```python
from build123d import *

# Parameters (mm, degrees)
F0_W     = 100
F0_H     = 200
F1_DEPTH = 30
F3_DEPTH = 10
F4_R     = 45
F4_R_2   = 5
F4_R_3   = 30
F5_DEPTH = 10
F6_DEPTH = 27
F7_DEPTH = 32
F9_DEPTH = 10


with BuildPart() as f1:
    # F0 (on Front) → F1 (new body)
    with BuildSketch(Plane.XZ):
        with Locations((50, -100)):
            Rectangle(F0_W, F0_H)
    extrude(amount=F1_DEPTH)

    # F2 (on face) → F3 (join)
    with BuildSketch(Plane(origin=(0, 0, 0), x_dir=(-1, 0, 0), z_dir=(0, 1, 0))):
        with BuildLine():
            ThreePointArc((-38.8196601125, -8.1037424163), (-43.876275643, -4.4106784786), (-50, -3.1037424163))
            ThreePointArc((-50, -3.1037424163), (-56.123724357, -4.4106784786), (-61.1803398875, -8.1037424163))
            Line((-61.1803398875, -8.1037424163), (-95.94427191, -46.971))
            ThreePointArc((-95.94427191, -46.971), (-98.2100683076, -50.6891349227), (-99, -54.971))
            Line((-99, -54.971), (-99, -138))
            ThreePointArc((-99, -138), (-96.0710678119, -145.0710678119), (-89, -148))
            Line((-89, -148), (-50, -148))
            Line((-50, -148), (-11, -148))
            ThreePointArc((-11, -148), (-3.9289321881, -145.0710678119), (-1, -138))
            Line((-1, -138), (-1, -54.971))
            ThreePointArc((-1, -54.971), (-1.7899316924, -50.6891349227), (-4.05572809, -46.971))
            Line((-4.05572809, -46.971), (-38.8196601125, -8.1037424163))
        make_face()
    extrude(amount=F3_DEPTH)

    # F4 (on face) → F5 (join)
    with BuildSketch(Plane(origin=(0, 10, 0), x_dir=(-1, 0, 0), z_dir=(0, 1, 0))):
        with Locations((-50, -98)):
            Circle(F4_R)
        with Locations((-50, -135.5)):
            Circle(F4_R_2, mode=Mode.SUBTRACT)
        with Locations((-87.5, -98)):
            Circle(F4_R_2, mode=Mode.SUBTRACT)
        with Locations((-50, -98)):
            Circle(F4_R_3, mode=Mode.SUBTRACT)
        with Locations((-12.5, -98)):
            Circle(F4_R_2, mode=Mode.SUBTRACT)
        with Locations((-50, -60.5)):
            Circle(F4_R_2, mode=Mode.SUBTRACT)
    extrude(amount=F5_DEPTH)

    # F6 (cut): faces of the model
    f6_faces = [f1.faces().sort_by_distance(p)[0] for p in [
        (50, 10, -135.5),
        (87.5, 10, -98),
        (50, 10, -60.5),
        (12.5, 10, -98),
    ]]
    extrude(f6_faces, amount=-F6_DEPTH, mode=Mode.SUBTRACT)

    # F7 (cut): a face of the model
    f7_faces = [f1.faces().sort_by_distance(p)[0] for p in [
        (50, 10, -98),
    ]]
    extrude(f7_faces, amount=-F7_DEPTH, mode=Mode.SUBTRACT)

    # F8 (on face) → F9 (cut)
    with BuildSketch(Plane(origin=(0, 0, 0), x_dir=(-1, 0, 0), z_dir=(0, 1, 0))):
        with BuildLine():
            ThreePointArc((-90, -177), (-86.4852813742, -185.4852813742), (-78, -189))
            Line((-78, -189), (-22, -189))
            ThreePointArc((-22, -189), (-13.5147186258, -185.4852813742), (-10, -177))
            Line((-10, -177), (-10, -171))
            ThreePointArc((-10, -171), (-13.5147186258, -162.5147186258), (-22, -159))
            Line((-22, -159), (-78, -159))
            ThreePointArc((-78, -159), (-86.4852813742, -162.5147186258), (-90, -171))
            Line((-90, -171), (-90, -177))
        make_face()
    extrude(amount=-F9_DEPTH, mode=Mode.SUBTRACT)


solid = f1.part
```
Part model, mm, in its own coordinate system. A direction names the side the tool comes from. Coordinates: 2 decimals unless noted, no trailing zeros. Loops run counter-clockwise (first coordinate to the right, second up) from the corner with the lowest first, then second, coordinate; pieces in that order, holes last. Notation, with made-up numbers: (-39, -31.5) - (-21, -31.5) arc R20 cw to (-21, -12.5) - close; hole circle Ø2 at (-6, -7). An arc over 180 degrees is marked (long way). Write item = value, one per line. Start each with the question number.
Item 1: Cut at B-B, the plane z = -98. Give the cut face in (x, y).
Item 2: Wall check: L1, parallel to Z at x = 50, y = 2; L2, parallel to Z at x = 50, y = -1; L3, parallel to Z at x = 12.5, y = -3.5. Give the ranges that are in metal, low to high. Write a range as from..to.
Item 3: Cut at C-C, the plane x = 34. Give the cut face in (y, z), and give its area (3 significant figures).
Item 4: Mould opens along Z. For faces 1 (the flat face through (51, 5, -148)), 2 (the cylindrical face through (13.58, 1.24, -102.88)), 3 (the cylindrical face through (72.111, -1.294, -77.725)), 4 (the flat face through (42, 0, -151)) say: released by +Z, released by -Z, zero draft, split by the parting line, or undercut.
Item 5: Cut at A-A, the plane y = -3. Give the cut face in (x, z).
Item 6: 3-axis set-ups, long thin cutter, end or side, ignore diameter. For faces 5 (the cylindrical face through (13.61, -4.93, -185.58)), 6 (the flat face through (1, 5, -97)), 7 (the flat face through (78.319, 4.93, -27.265)): which of +Z, -Z, +X, -X, +Y, -Y reach the whole face in a straight line?
Item 7: Cut at D-D, the plane z = -174. Give the cut face in (x, y).
Item 8: Flat gauge pins, fed straight in: pin 1 Ø8 at (x, z) = (48.5, -107) entering from +Y; pin 2 Ø1 at (y, z) = (4.5, -79.5) entering from +X; pin 3 Ø6 at (x, z) = (50, -135.5) entering from +Y. Where does each tip first touch, or does it go through?
The answers:
q1.outline = (0, -30) - (100, -30) - (100, 0) - (99, 0) - (99, 10) - (95, 10) - (95, 20) - (92.5, 20) - (92.5, -17) - (82.5, -17) - (82.5, 20) - (80, 20) - (80, -22) - (20, -22) - (20, 20) - (17.5, 20) - (17.5, -17) - (7.5, -17) - (7.5, 20) - (5, 20) - (5, 10) - (1, 10) - (1, 0) - (0, 0) - close
q2.L1 = -148..-140.5, -130.5..-128, -68..-65.5, -55.5..-3.1
q2.L2 = -200..-189, -159..-140.5, -130.5..-128, -68..-65.5, -55.5..0
q2.L3 = -200..-184.33, -163.67..-103, -93..0
q3.outline = (-30, -200) - (0, -200) - (0, -189) - (-10, -189) - (-10, -159) - (0, -159) - (0, -148) - (10, -148) - (10, -140.06) - (20, -140.06) - (20, -123.38) - (-22, -123.38) - (-22, -72.62) - (20, -72.62) - (20, -55.94) - (10, -55.94) - (10, -13.49) - (0, -13.49) - (0, 0) - (-30, 0) - close
q3.area = 5,750 mm2
q4.face_1 = released by -Z
q4.face_2 = undercut
q4.face_3 = undercut
q4.face_4 = zero draft
q5.outline = (0, -200) - (100, -200) - (100, 0) - (0, 0) - close; hole circle Ø10 at (12.5, -98); hole (10, -177) arc R12 ccw to (22, -189) - (78, -189) arc R12 ccw to (90, -177) - (90, -171) arc R12 ccw to (78, -159) - (22, -159) arc R12 ccw to (10, -171) - close; hole circle Ø60 at (50, -98); hole circle Ø10 at (50, -135.5); hole circle Ø10 at (50, -60.5); hole circle Ø10 at (87.5, -98)
q6.face_5 = +Y
q6.face_6 = +Z, -Z, -X, +Y
q6.face_7 = +Z, +X, +Y
q7.outline = (0, -30) - (100, -30) - (100, 0) - (90, 0) - (90, -10) - (10, -10) - (10, 0) - (0, 0) - close
q8.pin_1 = -22
q8.pin_2 = 99
q8.pin_3 = -17
